```python
from build123d import *

# Parameters (mm, degrees)
SKETCH1_R           = 18.93
SKETCH1_R_2         = 2.159
SKETCH1_R_3         = 2.5
SKETCH1_W           = 6.1
SKETCH1_H           = 24
BOSS_EXTRUDE1_DEPTH = 6.096


with BuildPart() as part:
    # Sketch1 → Boss-Extrude1 (new body)
    with BuildSketch(Plane(origin=(0, 0, 0), x_dir=(1, 0, 0), z_dir=(0, 1, 0))):
        with BuildLine():
            Line((-150, 120), (-10, 120))
            ThreePointArc((-10, 120), (-2.928932188, 117.071067812), (0, 110))
            Line((0, 110), (0, 0))
            Line((0, 0), (-32, 0))
            Line((-32, 0), (-32, 6.1))
            Line((-32, 6.1), (-64, 6.1))
            Line((-64, 6.1), (-64, 0))
            Line((-64, 0), (-96, 0))
            Line((-96, 0), (-96, 6.1))
            Line((-96, 6.1), (-128, 6.1))
            Line((-128, 6.1), (-128, 0))
            Line((-128, 0), (-160, 0))
            Line((-160, 0), (-160, 110))
            ThreePointArc((-160, 110), (-157.071067812, 117.071067812), (-150, 120))
        make_face()
        with Locations(Location((-108, 60, 0), (0, 0, 90))):
            Circle(SKETCH1_R, mode=Mode.SUBTRACT)
        with Locations(Location((-108, 91.089, 0), (0, 0, 90))):
            Circle(SKETCH1_R_2, mode=Mode.SUBTRACT)
        with Locations(Location((-81.076136222, 44.4555, 0), (0, 0, 90))):
            Circle(SKETCH1_R_2, mode=Mode.SUBTRACT)
        with Locations(Location((-134.923863778, 44.4555, 0), (0, 0, 90))):
            Circle(SKETCH1_R_2, mode=Mode.SUBTRACT)
        with Locations(Location((-48.1, 109.215, 0), (0, 0, 90))):
            Circle(SKETCH1_R_3, mode=Mode.SUBTRACT)
        with Locations(Location((-48.1, 10.785, 0), (0, 0, 90))):
            Circle(SKETCH1_R_3, mode=Mode.SUBTRACT)
        with Locations(Location((-10, 10.785, 0), (0, 0, 90))):
            Circle(SKETCH1_R_3, mode=Mode.SUBTRACT)
        with Locations(Location((-10, 109.215, 0), (0, 0, 90))):
            Circle(SKETCH1_R_3, mode=Mode.SUBTRACT)
        with Locations((-146.95, 84)):
            Rectangle(SKETCH1_W, SKETCH1_H, mode=Mode.SUBTRACT)
        with Locations((-146.95, 36)):
            Rectangle(SKETCH1_W, SKETCH1_H, mode=Mode.SUBTRACT)
        with Locations((-65.85, 84)):
            Rectangle(SKETCH1_W, SKETCH1_H, mode=Mode.SUBTRACT)
        with Locations((-65.85, 36)):
            Rectangle(SKETCH1_W, SKETCH1_H, mode=Mode.SUBTRACT)
        with Locations((-19.75, 36)):
            Rectangle(SKETCH1_W, SKETCH1_H, mode=Mode.SUBTRACT)
        with Locations((-19.75, 84)):
            Rectangle(SKETCH1_W, SKETCH1_H, mode=Mode.SUBTRACT)
    extrude(amount=BOSS_EXTRUDE1_DEPTH)


solid = part.part
```
For this review, take the finished solid that the model builds, in its own axes (mm). A direction names the side the tool comes from. Round coordinates to 2 decimals unless told otherwise and drop trailing zeros. Write each loop counter-clockwise with the first axis right and the second up, starting at its lowest first coordinate (ties: lowest second). Pieces come first, ordered by that corner, then holes. Notation, with made-up numbers: (-21.75, 19) -> (-1.75, 19) arc R34 cw to (-1.75, 54) -> close; hole circle Ø8 at (-17, 8). An arc over 180 degrees is marked (long way). One line per question, with ' | ' between items. Start each with the question number.
1) Add section A-A (x = -108). Write out the cut boundary in (y, z), and give its area (3 significant figures).
2) Mouldability with a two-part tool opening along Z and no side actions: class faces 1 (the cylindrical face through (-82.897, 3.005, -45.616)), 2 (the flat face through (-128, 3, -3)), 3 (the cylindrical face through (-3.01, 3.01, -117.15)) as +Z half, -Z half, draft (parallel to the pull), parting line (faces both ways), or undercut.
3) Add section C-C (z = -29). Write out the cut boundary in (x, y), and give its area (3 significant figures).
4) Add section D-D (x = -124). Write out the cut boundary in (y, z).
5) For pin 1 Ø3 at (x, y) = (-105, 3) entering from +Z, flat-tipped, find the tip position at first contact; note if it passes through.
6) Wall thickness on line 1 along X through (y, z) = (5.5, -5); line 2 along X through (y, z) = (2.25, -32.5); line 3 along Z through (x, y) = (-108, 4.75): over which ranges is each line inside the solid? List them lowest first.
7) Machinability: for faces 4 (the flat face through (-143.9, 3, -84)), 5 (the flat face through (-48, 3, -6.1)), 6 (the flat face through (-160, 3, -54)), which of the approach directions +Z, -Z, +X, -X, +Y, -Y give a long, thin tool a straight path to every point of the face, cutting with its end or side? Answer none if there is none.
8) Add section B-B (z = -60). Write out the cut boundary in (x, y).
Reported:
1) outline: (0, -120) -> (6.1, -120) -> (6.1, -93.25) -> (0, -93.25) -> close; (0, -88.93) -> (6.1, -88.93) -> (6.1, -78.93) -> (0, -78.93) -> close; (0, -41.07) -> (6.1, -41.07) -> (6.1, -6.1) -> (0, -6.1) -> close | area: 437 mm²
2) face 1: undercut | face 2: draft | face 3: -Z half
3) outline: (-160, 0) -> (-150, 0) -> (-150, 6.1) -> (-160, 6.1) -> close; (-143.9, 0) -> (-68.9, 0) -> (-68.9, 6.1) -> (-143.9, 6.1) -> close; (-62.8, 0) -> (-22.8, 0) -> (-22.8, 6.1) -> (-62.8, 6.1) -> close; (-16.7, 0) -> (0, 0) -> (0, 6.1) -> (-16.7, 6.1) -> close | area: 864 mm²
4) outline: (0, -120) -> (6.1, -120) -> (6.1, -70.12) -> (0, -70.12) -> close; (0, -49.88) -> (6.1, -49.88) -> (6.1, -6.1) -> (0, -6.1) -> close
5) pin 1: stops at z = -6.1
6) line 1: x = -160 to -128, -96 to -64, -32 to 0 | line 2: x = -160 to -150, -143.9 to -68.9, -62.8 to -22.8, -16.7 to 0 | line 3: z = -120 to -93.25, -88.93 to -78.93, -41.07 to -6.1
7) face 4: +Y, -Y | face 5: +Z, +Y, -Y | face 6: +Z, -Z, -X, +Y, -Y
8) outline: (-160, 0) -> (-126.93, 0) -> (-126.93, 6.1) -> (-160, 6.1) -> close; (-89.07, 0) -> (0, 0) -> (0, 6.1) -> (-89.07, 6.1) -> close
